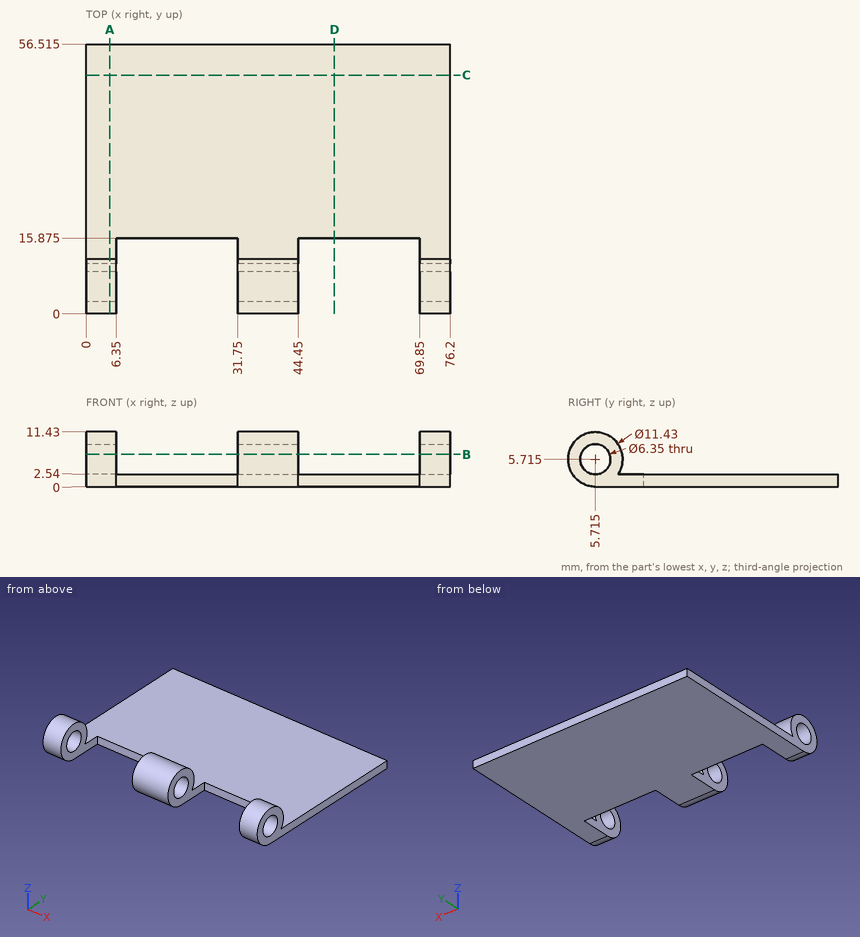
Answer from the drawing. Dimensions are ordinates in mm from the lowest x, y and z of the part. Coordinates: 2 decimals unless noted, no trailing zeros. Loops run counter-clockwise (first coordinate to the right, second up) from the corner with the lowest first, then second, coordinate; pieces in that order, holes last.
Q1. Each of these flat-tipped pins is pushed along its axis until it touches: pin 1 Ø3 at (x, z) = (62.5, 1.5) entering from -Y (3 decimals); pin 2 Ø6 at (y, z) = (32.5, 1.5) entering from -X; pin 3 Ø14 at (x, y) = (46, 40) entering from +Z; pin 4 Ø4 at (y, z) = (5.715, 5.715) entering from +X. Where does it stop, or does it pass through?
Q2. The part is cut by section D-D on x = 52. Write down the section's boundary in (y, z) (3 decimals).
Q3. The part is cut by section C-C on y = 50. Write down the section's boundary in (x, z).
Q4. The part is cut by section A-A on x = 5. Write down the section's boundary in (y, z) (3 decimals), and give its area (3 significant figures).
Q5. The part is cut by section B-B on z = 6.75. Write down the section's boundary in (x, y), and give its area (3 significant figures).
Q6. Consider probe 1 along X at (y, z) = (9, 6.5); probe 2 along Z at (x, y) = (30.5, 34); probe 3 along Y at (x, z) = (18, 2.5) (3 decimals). Determine where each line is inside the solid, lowest interval first.
Results below:
1. pin 1: stops at y = 15.875
1. pin 2: stops at x = 0
1. pin 3: stops at z = 2.54
1. pin 4: passes through
2. outline: (15.875, 0) - (56.515, 0) - (56.515, 2.54) - (15.875, 2.54) - close
3. outline: (0, 0) - (76.2, 0) - (76.2, 2.54) - (0, 2.54) - close
4. outline: (5.715, 0) - (56.515, 0) - (56.515, 2.54) - (10.467, 2.54) arc R5.715 ccw (long way) to start; hole circle Ø6.35 at (5.715, 5.715)
4. area: 191 mm2
5. outline: (0, 0.09) - (6.35, 0.09) - (6.35, 2.71) - (0, 2.71) - close; (0, 8.72) - (6.35, 8.72) - (6.35, 11.34) - (0, 11.34) - close; (31.75, 0.09) - (44.45, 0.09) - (44.45, 2.71) - (31.75, 2.71) - close; (31.75, 8.72) - (44.45, 8.72) - (44.45, 11.34) - (31.75, 11.34) - close; (69.85, 0.09) - (76.2, 0.09) - (76.2, 2.71) - (69.85, 2.71) - close; (69.85, 8.72) - (76.2, 8.72) - (76.2, 11.34) - (69.85, 11.34) - close
5. area: 133 mm2
6. probe 1: x = 0 to 6.35, 31.75 to 44.45, 69.85 to 76.2
6. probe 2: z = 0 to 2.54
6. probe 3: y = 15.875 to 56.515
